Autodesk Inventor part; units mm, degrees
ref_plane "YZ Plane" through (0, 0, 0) normal (1, 0, 0) x (0, 1, 0)
ref_plane "XZ Plane" through (0, 0, 0) normal (0, 1, 0) x (-1, 0, 0)
ref_plane "XY Plane" through (0, 0, 0) normal (0, 0, 1) x (1, 0, 0)
sketch "Sketch1" plane through (0, 0, 0) normal (0, 1, 0) x (-1, 0, 0)
  line L0 (0, 0) -> (-25.4, 0)
  line L1 (-25.4, 0) -> (-25.4, -3.175)
  line L2 (-25.4, -3.175) -> (0, -3.175)
  line L3 (0, -3.175) -> (0, 0)
  line L4 (-25.4, 0) -> (-22.225, 0)
  line L5 (-22.225, 0) -> (-22.225, -25.4)
  line L6 (-22.225, -25.4) -> (-25.4, -25.4)
  line L7 (-25.4, -25.4) -> (-25.4, 0)
  dimension "d0" = 25.4
  dimension "d1" = 3.175
  dimension "d2" = 25.4
  dimension "d3" = 3.175
extrude "Extrusion1" add sketch "Sketch1" along normal blind 101.6
sketch "Sketch2" plane through (25.4, 0, 0) normal (1, 0, 0) x (0, 0, -1)
  line L0 (0, 0) -> (0, 101.6)
  line L1 (0, 101.6) -> (12.7, 101.6)
  line L2 (25.4, 101.6) -> (3.175, 101.6)
  line L3 (12.7, 101.6) -> (12.7, 76.2)
  line L4 (0, 0) -> (12.7, 0)
  line L5 (0, 0) -> (25.4, 0)
  line L6 (12.7, 0) -> (12.7, 25.4)
  circle A0 centre (12.7, 76.2) radius 2.54
  circle A1 centre (12.7, 25.4) radius 2.54
  dimension "d6" = 12.7
  dimension "d7" = 25.4
  dimension "d8" = 25.4
  dimension "d9" = 5.08
extrude "Extrusion2" cut sketch "Sketch2" against normal blind 25.4
sketch "Sketch3" plane through (0, 0, 0) normal (0, 0, 1) x (1, 0, 0)
  line L0 (0, 0) -> (0, 101.6)
  line L1 (0, 0) -> (12.7, 0)
  line L2 (0, 0) -> (25.4, 0)
  line L3 (12.7, 0) -> (12.7, 25.4)
  line L4 (0, 101.6) -> (25.4, 101.6)
  line L5 (12.7, 101.6) -> (12.7, 76.2)
  circle A0 centre (12.7, 76.2) radius 2.54
  circle A1 centre (12.7, 25.4) radius 2.54
  dimension "d12" = 25.4
  dimension "d13" = 25.4
  dimension "d14" = 5.08
extrude "Extrusion3" cut sketch "Sketch3" against normal blind 25.4
properties part number "L Bracket 4in" material "Aluminum 6061"
CAD build for the part. Positions are in the model's coordinates, mm. A direction names the side the tool comes from. Round coordinates to 2 decimals unless told otherwise and drop trailing zeros. Write each loop counter-clockwise with the first axis right and the second up, starting at its lowest first coordinate (ties: lowest second). Pieces come first, ordered by that corner, then holes. Notation, with made-up numbers: (-11, -29.75) - (10, -29.75) arc R19 ccw to (10, -8.75) - close; hole circle Ø7 at (2, -16.75). An arc over 180 degrees is marked (long way). Write item = value, one per line. Start each with the question number.
Q1. Mould opens along X. For faces 1 (the cylindrical face through (12.15, 73.72, -1.57)), 2 (the cylindrical face through (23.83, 27.92, -12.37)), 3 (the flat face through (0, 50, -2)) say: pulls with the +X half, pulls with the -X half, needs draft (parallel to the pull), parting line crosses it, or undercut.
Q2. Which spindle directions (+Z, -Z, +X, -X, +Y, -Y) get a long thin tool onto all of the face, cutting with end or side? Do faces 4 (the flat face through (11, 50, -3.175)), 5 (the cylindrical face through (23.83, 73.72, -12.15)). Say none if no direction does.
Q3. Probe L1, parallel to Y at x = 22.95, z = -12.7; L2, parallel to X at y = 25.4, z = -1; L3, parallel to Z at x = 24.75, y = 25.4. List the from-to ranges inside material, lowest first. Write a range as from..to.
Q4. Band-saw the part on C-C (y = 76.2). Give the cut face in (x, z) (3 decimals).
Q5. Band-saw the part on A-A (z = -12.7). Give the cut face in (x, y) (3 decimals), then the cut area to 3 significant figures.
Q6. Drop flat-ended pins along their axis: pin 1 (11 mm diameter, centred on x = 9, y = 28.5, fed in from -Z) (3 decimals); pin 2 (6 mm diameter, centred on y = 76.2, z = -12.7, fed in from -X) (3 decimals). Give the stop position or say it passes through.
Q7. Band-saw the part on B-B (x = 12.7). Give the cut face in (y, z) (3 decimals).
Q8. Band-saw the part on D-D (y = 57.5). Give the cut face in (x, z) (3 decimals), then the cut area to 3 significant figures.
Answers below:
q1.face_1 = undercut
q1.face_2 = needs draft
q1.face_3 = pulls with the -X half
q2.face_4 = -Z, -X, +Y, -Y
q2.face_5 = +X, -X
q3.L1 = 0..22.86, 27.94..73.66, 78.74..101.6
q3.L2 = 0..10.16, 15.24..25.4
q3.L3 = -25.4..-15.24, -10.16..0
q4.outline = (0, -3.175) - (10.16, -3.175) - (10.16, 0) - (0, 0) - close; (15.24, -3.175) - (22.225, -3.175) - (22.225, -10.16) - (25.4, -10.16) - (25.4, 0) - (15.24, 0) - close; (22.225, -25.4) - (25.4, -25.4) - (25.4, -15.24) - (22.225, -15.24) - close
q5.outline = (22.225, 0) - (25.4, 0) - (25.4, 22.86) - (22.225, 22.86) - close; (22.225, 27.94) - (25.4, 27.94) - (25.4, 73.66) - (22.225, 73.66) - close; (22.225, 78.74) - (25.4, 78.74) - (25.4, 101.6) - (22.225, 101.6) - close
q5.area = 290 mm2
q6.pin_1 = -3.175
q6.pin_2 = 22.225
q7.outline = (0, -3.175) - (22.86, -3.175) - (22.86, 0) - (0, 0) - close; (27.94, -3.175) - (73.66, -3.175) - (73.66, 0) - (27.94, 0) - close; (78.74, -3.175) - (101.6, -3.175) - (101.6, 0) - (78.74, 0) - close
q8.outline = (0, -3.175) - (22.225, -3.175) - (22.225, -25.4) - (25.4, -25.4) - (25.4, 0) - (0, 0) - close
q8.area = 151 mm2
